Can you work these out from the model? Positions are in its coordinate system, mm. Face numbers are marked on the shaded views. A direction names the side the tool comes from. Give positions to 0.01 mm unless a question says otherwise; leave off trailing zeros. Loops run counter-clockwise (first coordinate to the right, second up) from the corner with the lowest first, then second, coordinate; pieces in that order, holes last. Notation, with made-up numbers: M 11,-16.75 L 63,-16.75 A34 ccw 63,17.25 Z; hole C 61,5 d6. An arc over 180 degrees is marked long. Answer as a JSON object with one key per item and string values.
```python
from build123d import *

# Parameters (mm, degrees)
SALIENTE_EXTRUIR1_DEPTH = 40
SALIENTE_EXTRUIR2_DEPTH = 5
SALIENTE_EXTRUIR3_DEPTH = 50
SALIENTE_EXTRUIR4_DEPTH = 14


with BuildPart() as part:
    # Croquis1 → Saliente-Extruir1 (new body)
    with BuildSketch(Plane.XY):
        with BuildLine():
            Line((0, 50), (0, 115))
            Line((0, 115), (-30, 115))
            Line((-30, 115), (-30, 120))
            Line((-30, 120), (5, 120))
            Line((5, 120), (5, 45))
            Line((5, 45), (0, 45))
            ThreePointArc((0, 45), (-45, 0), (0, -45))
            Line((0, -45), (5, -45))
            Line((5, -45), (5, -120))
            Line((5, -120), (-30, -120))
            Line((-30, -120), (-30, -115))
            Line((-30, -115), (0, -115))
            Line((0, -115), (0, -50))
            ThreePointArc((0, -50), (-50, 0), (0, 50))
        make_face()
    extrude(amount=SALIENTE_EXTRUIR1_DEPTH)

    # Croquis2 → Saliente-Extruir2 (add)
    with BuildSketch(Plane.XY.offset(40)):
        with BuildLine():
            Line((5, 120), (-30, 120))
            Line((-30, 120), (-30, 110))
            Line((-30, 110), (-5, 110))
            Line((-5, 110), (-5, 54.772255751))
            ThreePointArc((-5, 54.772255751), (-55, 0), (-5, -54.772255751))
            Line((-5, -54.772255751), (-5, -110))
            Line((-5, -110), (-30, -110))
            Line((-30, -110), (-30, -120))
            Line((-30, -120), (5, -120))
            Line((5, -120), (5, -45))
            Line((5, -45), (0, -45))
            ThreePointArc((0, -45), (-45, 0), (0, 45))
            Line((0, 45), (5, 45))
            Line((5, 45), (5, 120))
        make_face()
    saliente_extruir2 = extrude(amount=SALIENTE_EXTRUIR2_DEPTH)

    # Simetría1: Saliente-Extruir2 across plane
    add(saliente_extruir2.mirror(Plane.XY.offset(20)))

    # Croquis3 → Saliente-Extruir3 (add)
    with BuildSketch(Plane(origin=(0, 0, -5), x_dir=(-1, 0, 0), z_dir=(0, 0, -1))):
        with BuildLine():
            Line((-5, 45.111824995), (-5, 18.5))
            ThreePointArc((-5, 18.5), (13.5, 0), (-5, -18.5))
            Line((-5, -18.5), (-5, -44.72135955))
            Line((-5, -44.72135955), (-5, -45))
            Line((-5, -45), (0, -45))
            ThreePointArc((0, -45), (45, 0), (0, 45))
            Line((0, 45), (-5, 45.111824995))
        make_face()
    extrude(amount=-SALIENTE_EXTRUIR3_DEPTH)

    # Croquis4 → Saliente-Extruir4 (add)
    with BuildSketch(Plane(origin=(0, 0, -5), x_dir=(-1, 0, 0), z_dir=(0, 0, -1))):
        with BuildLine():
            Line((-5, 18.5), (-5, 16))
            ThreePointArc((-5, 16), (11, 0), (-5, -16))
            Line((-5, -16), (-5, -18.5))
            ThreePointArc((-5, -18.5), (13.5, 0), (-5, 18.5))
        make_face()
    saliente_extruir4 = extrude(amount=-SALIENTE_EXTRUIR4_DEPTH)

    # Simetría2: Saliente-Extruir4 across plane
    add(saliente_extruir4.mirror(Plane.XY.offset(20)))


solid = part.part
```
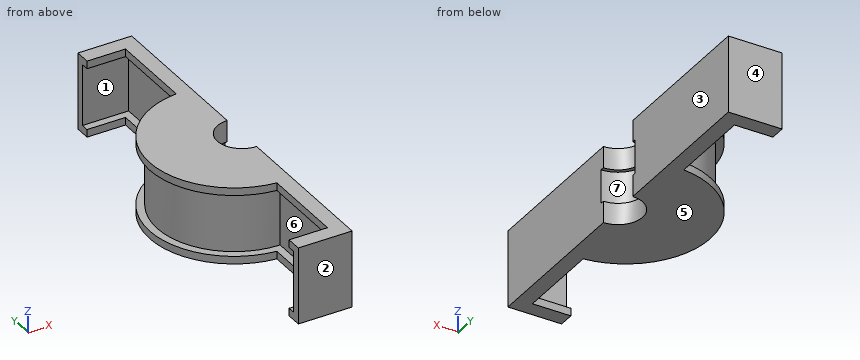
1) Will these pins go through, and if not, where does the flat tip stop? pin 1 Ø4 at (y, z) = (88, 43) entering from -X; pin 2 Ø11 at (y, z) = (-117.5, 13) entering from -X; pin 3 Ø4 at (x, y) = (-5.5, 61.5) entering from +Z; pin 4 Ø4 at (y, z) = (4, 32.5) entering from -X.
Answer list:
{"pin 1": "x = -5", "pin 2": "x = -30", "pin 3": "z = 45", "pin 4": "x = -49.96"}
2) Suppose I cut it at C-C, the plane z = 42.5. Write out the boundary of the cut face in (x, y), and give its area (3 significant figures).
Answer list:
{"outline": "M -30,-120 L 5,-120 L 5,-16 A16 cw 5,16 L 5,120 L -30,120 L -30,110 L -5,110 L -5,54.77 A55 ccw -5,-54.77 L -5,-110 L -30,-110 Z", "area": "6,700 mm^2"}
3) Suppose I cut it at B-B, the plane x = -18.5. Write out the boundary of the cut face in (y, z), and give its area (3 significant figures).
Answer list:
{"outline": "M -120,-5 L -110,-5 L -110,0 L -115,0 L -115,40 L -110,40 L -110,45 L -120,45 Z; M -51.8,-5 L 51.8,-5 L 51.8,0 L 46.45,0 L 46.45,40 L 51.8,40 L 51.8,45 L -51.8,45 L -51.8,40 L -46.45,40 L -46.45,0 L -51.8,0 Z; M 110,-5 L 120,-5 L 120,45 L 110,45 L 110,40 L 115,40 L 115,0 L 110,0 Z", "area": "5,350 mm^2"}
4) Please list where these lines run through material, in increasing order: line 1 along Y through (x, z) = (-24.5, 18); line 2 along Z through (x, y) = (-30, -45.5); line 3 along X through (y, z) = (67, -1). Write a range as from..to.
Answer list:
{"line 1": "-120..-115, -43.59..43.59, 115..120", "line 2": "-5..0, 40..45", "line 3": "-5..5"}
5) For the marked faces 5, 6 and 7, which set-ups out of +Z, -Z, +X, -X, +Y, -Y let a thin tool reach every point of the face, with its end or its side?
Answer list:
{"face 5": "-Z, +X, -X, +Y, -Y", "face 6": "-X", "face 7": "+X"}
6) Suppose I cut it at D-D, the plane x = -39. Write out the boundary of the cut face in (y, z).
Answer list:
{"outline": "M -38.78,-5 L 38.78,-5 L 38.78,0 L 31.29,0 L 31.29,40 L 38.78,40 L 38.78,45 L -38.78,45 L -38.78,40 L -31.29,40 L -31.29,0 L -38.78,0 Z"}
7) If we mould it in two halves opening along Y, with no side actions, what happens to the marked faces 1, 2, 3 and 4? For each: +Y half, -Y half, draft (parallel to the pull), parting line (faces both ways), or undercut.
Answer list:
{"face 1": "undercut", "face 2": "-Y half", "face 3": "draft", "face 4": "+Y half"}
8) Suppose I cut it at A-A, the plane y = 66. Write out the boundary of the cut face in (x, z), and give its area (3 significant figures).
Answer list:
{"outline": "M -5,-5 L 5,-5 L 5,45 L -5,45 L -5,40 L 0,40 L 0,0 L -5,0 Z", "area": "300 mm^2"}
